from build123d import *

# Parameters (mm, degrees)
SKETCH1_W           = 45
SKETCH1_H           = 40
BOSS_EXTRUDE1_DEPTH = 5
SKETCH2_R           = 12.7
CUT_EXTRUDE1_DEPTH  = 3.2
SKETCH3_W           = 4
SKETCH3_H           = 4
BOSS_EXTRUDE2_DEPTH = 55
SKETCH4_W           = 4
SKETCH4_H           = 4
BOSS_EXTRUDE3_DEPTH = 10
FILLET1_R           = 10
FILLET2_R           = 2
FILLET3_R           = 3
FILLET4_R           = 10


with BuildPart() as part:
    # Sketch1 → Boss-Extrude1 (new body)
    with BuildSketch(Plane(origin=(0, 0, 0), x_dir=(1, 0, 0), z_dir=(0, 1, 0))):
        Rectangle(SKETCH1_W, SKETCH1_H)
    extrude(amount=BOSS_EXTRUDE1_DEPTH)

    # Sketch2 → Cut-Extrude1 (cut)
    with BuildSketch(Plane(origin=(0, 0, 0), x_dir=(-1, 0, 0), z_dir=(0, -1, 0))):
        with Locations(Location((0, 0, 0), (0, 0, 90))):
            Circle(SKETCH2_R)
    extrude(amount=-CUT_EXTRUDE1_DEPTH, mode=Mode.SUBTRACT)

    # Sketch3 → Boss-Extrude2 (add)
    with BuildSketch(Plane(origin=(0, 5, 0), x_dir=(1, 0, 0), z_dir=(0, 1, 0))):
        with Locations((-20.5, -18)):
            Rectangle(SKETCH3_W, SKETCH3_H)
        with Locations((20.5, -18)):
            Rectangle(SKETCH3_W, SKETCH3_H)
    extrude(amount=BOSS_EXTRUDE2_DEPTH)

    # Sketch4 → Boss-Extrude3 (add)
    with BuildSketch(Plane(origin=(0, 0, 16), x_dir=(-1, 0, 0), z_dir=(0, 0, -1))):
        with Locations((20.5, 58)):
            Rectangle(SKETCH4_W, SKETCH4_H)
        with Locations((-20.5, 58)):
            Rectangle(SKETCH4_W, SKETCH4_H)
    extrude(amount=BOSS_EXTRUDE3_DEPTH)

    # Fillet1
    fillet1_edges = [part.edges().sort_by_distance(p)[0] for p in [
        (-18.5, 5, 18),
        (18.5, 5, 18),
    ]]
    fillet(fillet1_edges, radius=FILLET1_R)

    # Fillet2
    fillet2_edges = [part.edges().sort_by_distance(p)[0] for p in [
        (-20.5, 56, 16),
        (-20.5, 56, 6),
        (20.5, 56, 16),
        (20.5, 56, 6),
    ]]
    fillet(fillet2_edges, radius=FILLET2_R)

    # Fillet3
    fillet3_edges = [part.edges().sort_by_distance(p)[0] for p in [
        (-15.5, 5, 16),
        (15.5, 5, 16),
    ]]
    fillet(fillet3_edges, radius=FILLET3_R)

    # Fillet4
    fillet4_edges = [part.edges().sort_by_distance(p)[0] for p in [
        (-22.5, 2.5, -20),
        (22.5, 2.5, -20),
    ]]
    fillet(fillet4_edges, radius=FILLET4_R)


solid = part.part
Input: part model. Units: mm. Frame: model coordinates. A direction names the side the tool comes from. Give positions to 0.01 mm unless a question says otherwise; leave off trailing zeros. Order: outer loops, then holes, each group sorted by start corner. A loop starts at its lowest first (then second) coordinate and runs counter-clockwise, first axis right, second up. Notation, with made-up numbers: M -8,-1 L -3,-1 A19 cw -3,36 Z; hole C -15,44 d4. An arc over 180 degrees is marked long. Answer as a JSON object with one key per item and string values.
1. Cut plane C-C, the plane y = 24. Output: boundary loops of the cut face in (x, z), and give its area (3 significant figures).
Result sheet:
{"outline": "M -22.5,16 L -18.5,16 L -18.5,20 L -22.5,20 Z; M 18.5,16 L 22.5,16 L 22.5,20 L 18.5,20 Z", "area": "32.0 mm²"}
2. Cut plane A-A, the plane z = 0. Output: boundary loops of the cut face in (x, y), and give its area (3 significant figures).
Result sheet:
{"outline": "M -22.5,0 L -12.7,0 L -12.7,3.2 L 12.7,3.2 L 12.7,0 L 22.5,0 L 22.5,5 L -22.5,5 Z", "area": "144 mm²"}
3. Cut plane D-D, the plane z = 7. Output: boundary loops of the cut face in (x, y).
Result sheet:
{"outline": "M -22.5,0 L -10.6,0 L -10.6,3.2 L 10.6,3.2 L 10.6,0 L 22.5,0 L 22.5,5 L -22.5,5 Z; M -22.5,56.27 L -18.5,56.27 L -18.5,60 L -22.5,60 Z; M 18.5,56.27 L 22.5,56.27 L 22.5,60 L 18.5,60 Z"}
4. Pull-direction query (X, two-part tool) for faces 1 (the flat face through (-18.5, 42.2, 16.2)), 2 (the flat face through (21, 59, 6)), 3 (the flat face through (22.5, 25.4, 16.2)), 4 (the cylindrical face through (-7.7, 1.6, 10.1)); classes: +X half, -X half, draft (parallel to the pull), parting line (faces both ways), or undercut.
Result sheet:
{"face 1": "undercut", "face 2": "draft", "face 3": "+X half", "face 4": "undercut"}
5. Reachability of faces 5 (the cylindrical face through (20.47, 56.57, 6.6)), 6 (the cylindrical face through (15.65, 8.01, 18.01)), 7 (the flat face through (-20, 59, 6)), 8 (the flat face through (20, 60, 13)), 9 (the flat face through (0, 3.2, 0)) from +Z, -Z, +X, -X, +Y, -Y: full face, straight path, thin tool, end or side. Return the list, or none.
Result sheet:
{"face 5": "-Z, +X, -X", "face 6": "+Z, -Z, +Y", "face 7": "-Z, +X, -X, +Y", "face 8": "+Z, -Z, +X, -X, +Y", "face 9": "-Y"}
6. Ray query, line 1 (X direction, y = 1.8, z = 0); line 2 (Y direction, x = 4, z = 1.5); line 3 (Y direction, x = -15, z = -11). Return the intervals inside material, ascending. Write a range as [from, to].
Result sheet:
{"line 1": "[-22.5, -12.7], [12.7, 22.5]", "line 2": "[3.2, 5]", "line 3": "[0, 5]"}
7. Cut plane B-B, the plane x = 0. Output: boundary loops of the cut face in (y, z), and give its area (3 significant figures).
Result sheet:
{"outline": "M 0,-20 L 5,-20 L 5,20 L 0,20 L 0,12.7 L 3.2,12.7 L 3.2,-12.7 L 0,-12.7 Z", "area": "119 mm²"}
8. First-contact query: P1, Ø4, axis at x = -1, z = 10.5, coming from the +Y side; P2, Ø3, axis at x = 16.5, y = 23.5, coming from the -Z side; P3, Ø1, axis at x = -20.5, y = 58.5, coming from the -Z side; P4, Ø7.5, axis at x = 20.5, y = 25, coming from the -Z side. Flat tips, straight axial feed; report the tip coordinate or a pass-through.
Result sheet:
{"P1": "y = 5", "P2": "through", "P3": "z = 6", "P4": "z = 16"}
